Source: CAD feature listing. Evaluate the final solid. Frame: model axes, mm. A direction names the side the tool comes from. Give positions to 0.01 mm unless a question says otherwise; leave off trailing zeros. Write each loop counter-clockwise with the first axis right and the second up, starting at its lowest first coordinate (ties: lowest second). Pieces come first, ordered by that corner, then holes. Notation, with made-up numbers: (67, 17.5) -> (112, 17.5) arc R20 cw to (112, 32.5) -> close; hole circle Ø2 at (-33.5, 3). An arc over 180 degrees is marked (long way). Answer as a JSON object with one key per item and string values. Group by question number.
Item 1: Pull-direction query (Y, two-part tool) for faces 4 (the face through (32, -39, 36)), 5 (the face through (30, 100.5, 18)), 6 (the face through (32, -77.5, 17)); classes: pulls with the +Y half, pulls with the -Y half, needs draft (parallel to the pull), parting line crosses it, or undercut.
Item 2: First-contact query: pin 1 Ø1.5 at (y, z) = (6, 1) entering from +X; pin 2 Ø2.5 at (y, z) = (8, 1) entering from -X; pin 3 Ø2 at (x, y) = (-10.5, -10.5) entering from -Z. Flat tips, straight axial feed; report the tip coordinate or a pass-through.
Item 3: Section query A-A on z = 28. Return the cut outline in (x, y).
Item 4: Ray query, probe 1 along Y at (x, z) = (54, 22); probe 2 along X at (y, z) = (89.5, 10.5); probe 3 along Y at (x, z) = (-45.5, 23.5). Return the intervals inside material, ascending. Write a range as from..to.
Item 5: Section query B-B on x = -20. Return the cut outline in (y, z).
Item 6: Access query for faces 1 (the face through (-47, 33, 18)), 2 (the face through (55, 11, 3)), 3 (the face through (32, -39, 34)). Directions: +Z, -Z, +X, -X, +Y, -Y. A direction counts if a zero-diameter tool reaches every point of the face in a straight line with its end or side. Return the directions, or none.
Item 7: Section query C-C on y = 57.5. Return the cut outline in (x, z).
Item 8: Section query D-D on x = 90.5. Return the cut outline in (y, z).
from build123d import *

# Parameters (mm, degrees)
SKETCH_W     = 121
SKETCH_H     = 21
PAD_DEPTH    = 3
PAD001_DEPTH = 34
PAD002_DEPTH = 2
SKETCH003_W  = 10
SKETCH003_H  = 21
POCKET_DEPTH = 36.001


with BuildPart() as part:
    # Sketch → Pad (new body)
    with BuildSketch(Plane.XY):
        with Locations((60.5, 10.5)):
            Rectangle(SKETCH_W, SKETCH_H)
    extrude(amount=PAD_DEPTH)

    # Sketch001 (on Face5 of Pad) → Pad001 (join)
    with BuildSketch(Plane(origin=(0, 0, 0), x_dir=(1, 0, 0), z_dir=(0, 0, -1))):
        Polygon((121, -100.5), (121, -21), (-35, -21), (-59, -45), (-59, -100.5), align=None)
        Polygon((119, -98.5), (119, -23), (-34.171573, -23), (-57, -45.828427), (-57, -98.5), align=None, mode=Mode.SUBTRACT)
        Polygon((121, 0), (-35, 0), (-59, 24), (-59, 79.5), (121, 79.5), align=None)
        Polygon((-57, 77.5), (-57, 24.828427), (-34.171573, 2), (119, 2), (119, 77.5), align=None, mode=Mode.SUBTRACT)
    extrude(amount=-PAD001_DEPTH)

    # Sketch002 (on Face3 of Pad001) → Pad002 (join)
    with BuildSketch(Plane.XY.offset(34)):
        Polygon((-59, -79.5), (-59, -24), (-35, 0), (121, 0), (121, -79.5), align=None)
        Polygon((-35, 21), (-59, 45), (-59, 100.5), (121, 100.5), (121, 21), align=None)
    extrude(amount=PAD002_DEPTH)

    # Sketch003 (on Face5 of Pad002) → Pocket (cut, through all)
    with BuildSketch(Plane(origin=(0, 0, 0), x_dir=(1, 0, 0), z_dir=(0, 0, -1))):
        with Locations((116, -10.5)):
            Rectangle(SKETCH003_W, SKETCH003_H)
    extrude(amount=-POCKET_DEPTH, mode=Mode.SUBTRACT)


solid = part.part
Worked answers:
{
 "1": {"face 4": "needs draft", "face 5": "pulls with the +Y half", "face 6": "undercut"},
 "2": {"pin 1": "x = 111", "pin 2": "x = 0", "pin 3": "z = 34"},
 "3": {"outline": "(-59, -79.5) -> (121, -79.5) -> (121, 0) -> (-35, 0) -> (-59, -24) -> close; (-59, 45) -> (-35, 21) -> (121, 21) -> (121, 100.5) -> (-59, 100.5) -> close; hole (-57, -77.5) -> (119, -77.5) -> (119, -2) -> (-34.17, -2) -> (-57, -24.83) -> close; hole (-57, 45.83) -> (-34.17, 23) -> (119, 23) -> (119, 98.5) -> (-57, 98.5) -> close"},
 "4": {"probe 1": "-79.5..-77.5, -2..0, 21..23, 98.5..100.5", "probe 2": "-59..-57, 119..121", "probe 3": "-79.5..-77.5, -13.33..-10.5, 31.5..34.33, 98.5..100.5"},
 "5": {"outline": "(-79.5, 0) -> (-77.5, 0) -> (-77.5, 34) -> (-2, 34) -> (-2, 0) -> (0, 0) -> (0, 36) -> (-79.5, 36) -> close; (21, 0) -> (23, 0) -> (23, 34) -> (98.5, 34) -> (98.5, 0) -> (100.5, 0) -> (100.5, 36) -> (21, 36) -> close"},
 "6": {"face 1": "+Z, -Z, -X", "face 2": "+Z, +X, -X", "face 3": "-Z"},
 "7": {"outline": "(-59, 0) -> (-57, 0) -> (-57, 34) -> (119, 34) -> (119, 0) -> (121, 0) -> (121, 36) -> (-59, 36) -> close"},
 "8": {"outline": "(-79.5, 0) -> (-77.5, 0) -> (-77.5, 34) -> (-2, 34) -> (-2, 0) -> (23, 0) -> (23, 34) -> (98.5, 34) -> (98.5, 0) -> (100.5, 0) -> (100.5, 36) -> (21, 36) -> (21, 3) -> (0, 3) -> (0, 36) -> (-79.5, 36) -> close"}
}
